```python
from build123d import *

# Parameters (mm, degrees)
F0_W     = 350
F0_H     = 350
F0_R     = 6.35
F0_W_2   = 250
F0_H_2   = 250
F1_DEPTH = 19.05
F2_R     = 50
F3_R     = 3.175
F4_DEPTH = 25


with BuildPart() as f1:
    # F0 (on Front) → F1 (new body)
    with BuildSketch(Plane.XZ):
        with Locations((175, 175)):
            Rectangle(F0_W, F0_H)
        with Locations((20, 20)):
            Circle(F0_R, mode=Mode.SUBTRACT)
        with Locations((330, 20)):
            Circle(F0_R, mode=Mode.SUBTRACT)
        with Locations((175, 175)):
            Rectangle(F0_W_2, F0_H_2, mode=Mode.SUBTRACT)
    extrude(amount=F1_DEPTH)

    # F2
    f2_edges = [f1.edges().sort_by_distance(p)[0] for p in [
        (300, -9.525, 50),
        (300, -9.525, 300),
        (50, -9.525, 300),
        (50, -9.525, 50),
        (350, -9.525, 350),
    ]]
    fillet(f2_edges, radius=F2_R)

    # F3 (on face) → F4 (cut)
    with BuildSketch(Plane.XZ.offset(19.05)):
        with Locations((25, 275)):
            Circle(F3_R)
        with Locations((25, 75)):
            Circle(F3_R)
    extrude(amount=-F4_DEPTH, mode=Mode.SUBTRACT)


solid = f1.part
```
Read the model definition and answer for the solid it produces. Units are mm, in the model's axes. A direction names the side the tool comes from. Round coordinates to 2 decimals unless told otherwise and drop trailing zeros. Write each loop counter-clockwise with the first axis right and the second up, starting at its lowest first coordinate (ties: lowest second). Pieces come first, ordered by that corner, then holes. Notation, with made-up numbers: (53, -34.75) - (79, -34.75) arc R8 ccw to (79, -29.75) - close; hole circle Ø7 at (13, 4.25). An arc over 180 degrees is marked (long way). Use CSV: the item, a comma, the result in double quotes.
Q1. Determine the mould class of faces 1 (the flat face through (148, -9, 350)), 2 (the flat face through (174, -9, 300)), 3 (the cylindrical face through (65.036, -9.658, 64.258)), 4 (the flat face through (350, -9, 148)) for opening direction X: +X half, -X half, draft (parallel to the pull), parting line (faces both ways), or undercut.
Values:
face 1,"draft"
face 2,"undercut"
face 3,"undercut"
face 4,"+X half"
Q2. Find section D-D, the plane z = 324. Write down the section's boundary in (x, y).
Values:
outline,"(0, -19.05) - (343.86, -19.05) - (343.86, 0) - (0, 0) - close"
Q3. Each of these flat-tipped pins is pushed along its axis until it touches: pin 1 Ø14.5 at (x, z) = (20, 20) entering from +Y; pin 2 Ø4 at (x, z) = (25, 75) entering from +Y. Where does it stop, or does it pass through?
Values:
pin 1,"stops at y = 0"
pin 2,"passes through"
Q4. Find section B-B, the plane z = 206. Write down the section's boundary in (x, y), then the cut area to 4 significant figures.
Values:
outline,"(0, -19.05) - (50, -19.05) - (50, 0) - (0, 0) - close; (300, -19.05) - (350, -19.05) - (350, 0) - (300, 0) - close"
area,"1,905 mm²"
Q5. Find section A-A, the plane x = 330. Write down the section's boundary in (y, z).
Values:
outline,"(-19.05, 0) - (0, 0) - (0, 13.65) - (-19.05, 13.65) - close; (-19.05, 26.35) - (0, 26.35) - (0, 340) - (-19.05, 340) - close"
Q6. A tool of negligible diameter and unlimited length cuts with its end or side. For faces 5 (the cylindrical face through (65.036, -9.658, 285.742)), 6 (the flat face through (173, -9, 0)), from which of +Z, -Z, +X, -X, +Y, -Y can it reach the whole face along a straight path? Write none if from no direction.
Values:
face 5,"+Y, -Y"
face 6,"-Z, +X, -X, +Y, -Y"
Q7. Straight lines are drawn through the part: line 1 along X through (y, z) = (-2.5, 99); line 2 along Z through (x, y) = (154, -4); line 3 along Z through (x, y) = (25, -14) (3 decimals). For each, find the intervals that lie inside material, in ascending order.
Values:
line 1,"x = 0 to 50.01, 299.99 to 350"
line 2,"z = 0 to 50, 300 to 350"
line 3,"z = 0 to 16.086, 23.914 to 71.825, 78.175 to 271.825, 278.175 to 350"
Q8. Find section C-C, the plane y = -11.5. Write down the section's boundary in (x, z) (3 decimals), then the cut area to 3 significant figures.
Values:
outline,"(0, 0) - (350, 0) - (350, 300) arc R50 ccw to (300, 350) - (0, 350) - close; hole circle Ø12.7 at (20, 20); hole circle Ø6.35 at (25, 75); hole circle Ø6.35 at (25, 275); hole (50, 100) arc R50 ccw to (100, 50) - (250, 50) arc R50 ccw to (300, 100) - (300, 250) arc R50 ccw to (250, 300) - (100, 300) arc R50 ccw to (50, 250) - close; hole circle Ø12.7 at (330, 20)"
area,"61,300 mm²"
